Could you check a few things on this drawing? It's one solid part, dimensions in mm from its lowest x, y, z. A direction names the side the tool comes from. Coordinates: 2 decimals unless noted, no trailing zeros. Write each loop counter-clockwise with the first axis right and the second up, starting at its lowest first coordinate (ties: lowest second). Pieces come first, ordered by that corner, then holes.
Item 1: I want a section at D-D (x = 21.5). Please give me the cut outline in (y, z), and give its area (3 significant figures).
Item 2: Please list where these lines run through material, in increasing order: line 1 (X direction, y = 38.1, z = 30.25); line 2 (Y direction, x = 76, z = 27) (1 decimal); line 3 (X direction, y = 13.5, z = 40).
Item 3: For the marked faces 1, 2 and 3, which set-ups out of +Z, -Z, +X, -X, +Y, -Y let a thin tool reach every point of the face, with its end or its side?
Item 4: I'm going to push flat-ended pins straight in: P1, Ø7.5, axis at y = 11.5, z = 56, coming from the +X side; P2, Ø6, axis at x = 42.86, y = 19.65, coming from the +Z side; P3, Ø10.5, axis at y = 12.5, z = 46.5, coming from the -X side. Where does each tip first touch, or does it pass through?
Item 5: I want a section at C-C (x = 63). Please give me the cut outline in (y, z), and give its area (3 significant figures).
Item 6: I want a section at B-B (y = 28.5). Please give me the cut outline in (x, z), and give its area (3 significant figures).
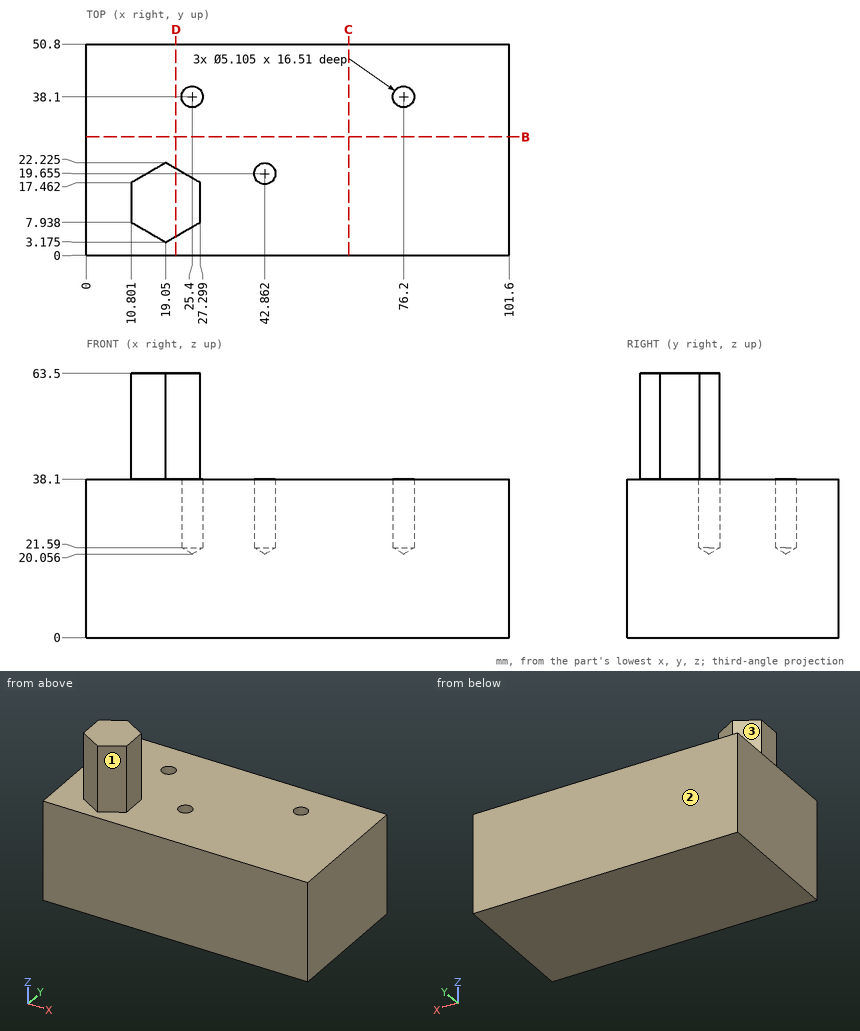
Answer:
1. outline: (0, 0) - (50.8, 0) - (50.8, 38.1) - (20.81, 38.1) - (20.81, 63.5) - (4.59, 63.5) - (4.59, 38.1) - (0, 38.1) - close
1. area: 2,350 mm2
2. line 1: x = 0 to 22.85, 27.95 to 73.65, 78.75 to 101.6
2. line 2: y = 0 to 35.6, 40.6 to 50.8
2. line 3: x = 10.8 to 27.3
3. face 1: +Z, +X, -Y
3. face 2: +Z, -Z, +X, -X, +Y
3. face 3: +Z, -X, +Y
4. P1: stops at x = 27.3
4. P2: stops at z = 38.1
4. P3: stops at x = 10.8
5. outline: (0, 0) - (50.8, 0) - (50.8, 38.1) - (0, 38.1) - close
5. area: 1,940 mm2
6. outline: (0, 0) - (101.6, 0) - (101.6, 38.1) - (0, 38.1) - close
6. area: 3,870 mm2
